```python
from build123d import *

# Parameters (mm, degrees)
F0_R     = 1.5
F1_DEPTH = 3
F2_R     = 32.5
F3_DEPTH = 3
F5_R     = 2
F6_DEPTH = 3


with BuildPart() as f1:
    # F0 (on Front) → F1 (new body)
    with BuildSketch(Plane.XZ):
        Polygon((102, 117), (102, 120), (62, 120), (62, 117), (19, 117), (19, 120), (-21, 120), (-21, 117), (-64, 117), (-64, 120), (-104, 120), (-104, 117), (-177, 117), (-177, -115), (-152, -115), (-152, -95), (-102, -95), (-102, -120), (160, -120), (160, -115), (176, -115), (176, 117), align=None)
        with Locations((-161, -104)):
            Circle(F0_R, mode=Mode.SUBTRACT)
        with Locations((160, -104)):
            Circle(F0_R, mode=Mode.SUBTRACT)
        with Locations((-161, 104)):
            Circle(F0_R, mode=Mode.SUBTRACT)
        with Locations((160, 104)):
            Circle(F0_R, mode=Mode.SUBTRACT)
    extrude(amount=F1_DEPTH)

    # F2 (on face) → F3 (cut)
    with BuildSketch(Plane(origin=(0, 0, 0), x_dir=(-1, 0, 0), z_dir=(0, 1, 0))):
        with Locations((0, 54.959509)):
            Circle(F2_R)
    extrude(amount=-F3_DEPTH, mode=Mode.SUBTRACT)

    # F5 (on face) → F6 (cut)
    with BuildSketch(Plane(origin=(0, 0, 0), x_dir=(-1, 0, 0), z_dir=(0, 1, 0))):
        with Locations((-30.492457, 85.465)):
            Circle(F5_R)
        with Locations((31.007543, 85.464843)):
            Circle(F5_R)
        with Locations((30.500002, 23.964843)):
            Circle(F5_R)
        with Locations((-30.999998, 23.965)):
            Circle(F5_R)
    extrude(amount=-F6_DEPTH, mode=Mode.SUBTRACT)


solid = f1.part
```
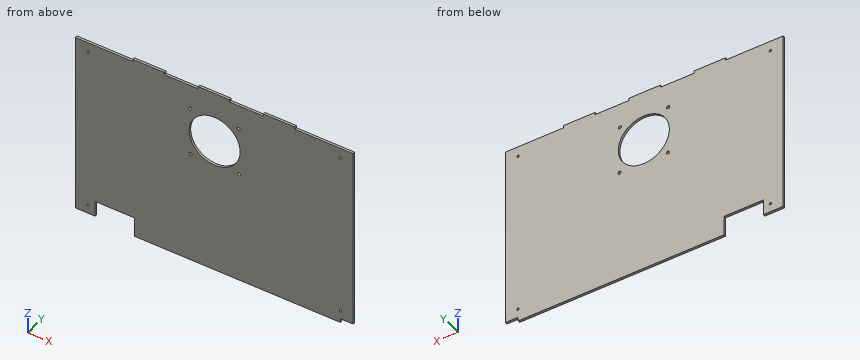
Source: CAD feature listing. Evaluate the final solid. Frame: model axes, mm. Coordinates: 2 decimals unless noted, no trailing zeros. Write each loop counter-clockwise with the first axis right and the second up, starting at its lowest first coordinate (ties: lowest second). Pieces come first, ordered by that corner, then holes. Notation, with made-up numbers: M -31,-12 L 3,-12 A25 ccw 3,7 Z; hole C 75.25,89.25 d8. An arc over 180 degrees is marked long. Answer as a JSON object with one key per item and string values.
1. Cut plane C-C on y = -2.2. State how many separate pieces and enclosed holes the cut face has, plus the area to 3 significant figures.
Evaluation:
{"separate pieces": "1", "enclosed holes": "9", "area": "79,200 mm^2"}
2. Cut plane B-B on x = 0. Output: boundary loops of the cut face in (y, z).
Evaluation:
{"outline": "M -3,-120 L 0,-120 L 0,22.46 L -3,22.46 Z; M -3,87.46 L 0,87.46 L 0,120 L -3,120 Z"}
3. Cut plane A-A on z = 63.5. Output: boundary loops of the cut face in (x, y).
Evaluation:
{"outline": "M -177,-3 L -31.36,-3 L -31.36,0 L -177,0 Z; M 31.36,-3 L 176,-3 L 176,0 L 31.36,0 Z"}
4. Contact query for flat-ended pins moving along their axis: P1, Ø1.5, axis at y = -1.5, z = 118.5, coming from the -X side; P2, Ø1.5, axis at y = -2, z = 118.5, coming from the +X side; P3, Ø1.5, axis at x = -38.5, y = -2, coming from the +Z side; P4, Ø1.8, axis at x = -161, z = -104, coming from the +Y side. Output: stop coordinate, or through.
Evaluation:
{"P1": "x = -104", "P2": "x = 102", "P3": "z = 117", "P4": "through"}
5. Ray query, L1, parallel to Z at x = -161, y = -1.7; L2, parallel to X at y = -2, z = -104; L3, parallel to Z at x = 38.5, y = -0.5. Return the intervals inside material, ascending.
Evaluation:
{"L1": "-115 to -105.5, -102.5 to 102.5, 105.5 to 117", "L2": "-177 to -162.5, -159.5 to -152, -102 to 158.5, 161.5 to 176", "L3": "-120 to 117"}
